Part print with two shaded views. Sizes in mm from the minimum x, y, z corner. Give positions to 0.01 mm unless a question says otherwise; leave off trailing zeros. Order: outer loops, then holes, each group sorted by start corner. A loop starts at its lowest first (then second) coordinate and runs counter-clockwise, first axis right, second up.
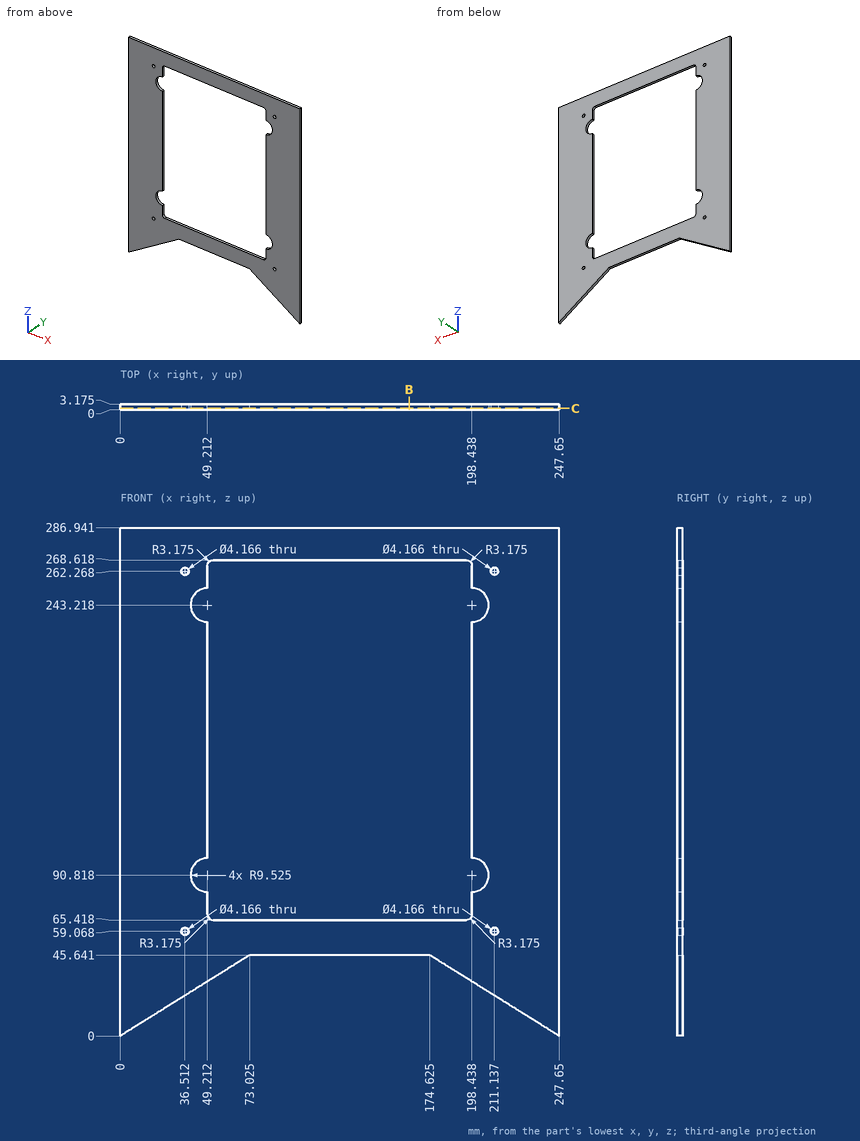
1. Wall check: line 1 (Z direction, x = 83, y = 2.3); line 2 (X direction, y = 0.15, z = 200.5). Give the ranges that are in metal, low to high.
2. Saw through at C-C on y = 0.65. State how many separate pieces and enclosed holes the cut face has, plus the area to 3 significant figures.
3. Pin check, flat tips, straight feed: P1, Ø3.5, axis at x = 211.14, z = 262.27, coming from the -Y side; P2, Ø1.6, axis at x = 128.5, y = 2.5, coming from the -Z side. Stop position of each tip, or through.
4. Saw through at B-B on x = 163. Give the cut face in (y, z) (1 decimal).
Reported:
1. line 1: z = 45.64 to 65.42, 268.62 to 286.94
1. line 2: x = 0 to 49.21, 198.44 to 247.65
2. separate pieces: 1
2. enclosed holes: 5
2. area: 32,200 mm2
3. P1: passes through
3. P2: stops at z = 45.64
4. outline: (0, 45.6) - (3.2, 45.6) - (3.2, 65.4) - (0, 65.4) - close; (0, 268.6) - (3.2, 268.6) - (3.2, 286.9) - (0, 286.9) - close
